CAD build for the part. Positions are in the model's coordinates, mm. A direction names the side the tool comes from. Give positions to 0.01 mm unless a question says otherwise; leave off trailing zeros. Write each loop counter-clockwise with the first axis right and the second up, starting at its lowest first coordinate (ties: lowest second). Pieces come first, ordered by that corner, then holes. Notation, with made-up numbers: (69, 39.25) -> (118, 39.25) arc R21 cw to (118, 46.25) -> close; hole circle Ø11 at (25, 36.5). An arc over 180 degrees is marked (long way). Answer in a Markdown table with one row per item. Add a question column.
```python
from build123d import *

# Parameters (mm, degrees)
BASE_EXTRUDE_DEPTH     = 3.81
SKETCHED_START         = -15.875
SKETCHED_BEND1_DEPTH   = 31.75
SKETCHED_BEND1_2_DEPTH = 31.75


# Read off the part's stored shape, not the designer's step: Sketched Bend1
with BuildPart() as part:
    # Sketch1 → Base-Extrude (new body)
    with BuildSketch(Plane.XY):
        with BuildLine():
            Line((15.875, 68.022105782), (15.875, 254))
            Line((15.875, 254), (-15.875, 254))
            Line((-15.875, 254), (-15.875, 68.022105782))
            ThreePointArc((-15.875, 68.022105782), (0, -69.85), (15.875, 68.022105782))
        make_face()
    extrude(amount=BASE_EXTRUDE_DEPTH)

    # Sketched Bend1 outline → Sketched Bend1 (cut)
    with BuildSketch(Plane.YZ.offset(SKETCHED_START)):
        with BuildLine():
            ThreePointArc((121.7921973, 3.81), (127.40036545, 2.828314461), (132.341609606, 0))
            Line((132.341609606, 0), (254, 0))
            Line((254, 0), (254, 3.81))
            Line((254, 3.81), (121.7921973, 3.81))
        make_face()
    extrude(amount=SKETCHED_BEND1_DEPTH, mode=Mode.SUBTRACT)

    # Sketched Bend1 2 outline → Sketched Bend1 2 (add)
    with BuildSketch(Plane.YZ.offset(SKETCHED_START)):
        with BuildLine():
            Line((123.653365296, -25.262883972), (35.007053077, -38.395670967))
            Line((35.007053077, -38.395670967), (35.565403476, -42.164536159))
            Line((35.565403476, -42.164536159), (124.211715695, -29.031749163))
            ThreePointArc((124.211715695, -29.031749163), (137.690590482, -17.152099982), (132.341609606, 0))
            Line((132.341609606, 0), (121.7921973, 0))
            ThreePointArc((121.7921973, 0), (134.457871906, -11.766894015), (123.653365296, -25.262883972))
        make_face()
    extrude(amount=SKETCHED_BEND1_2_DEPTH)


solid = part.part
```
Item 1: Slice it at C-C, the plane z = -17. List the corners of the cut face in (x, y) (3 decimals), then the cut area to 3 significant figures.
Item 2: Probe L1, parallel to Z at x = 28.5, y = 5.5; L2, parallel to Z at x = -14, y = 50.5; L3, parallel to Z at x = 2.5, y = 73.5. List the from-to ranges inside material, lowest first. Write a range as from..to.
Item 3: Mould opens along Z. For faces 4 (the face through (-0.22, 79.27, -35.69)), 5 (the face through (-0.222, 134.436, -11.502)), 6 (the face through (15.875, 102, -29)) say: released by +Z, released by -Z, zero draft, split by the parting line, or undercut.
Item 4: Slice it at D-D, the plane y = 0. List the corners of the cut face in (x, z).
Item 5: Which spindle directions (+Z, -Z, +X, -X, +Y, -Y) get a long thin tool onto all of the face, cutting with end or side? Do faces 1 (the face through (-15.875, 102, -29)), 2 (the face through (-1, 6, 3.81)), 3 (the face through (-1, 6, 0)). Say none if no direction does.
Item 6: Slice it at A-A, the plane y = 93.5. List the corners of the cut face in (x, z) (3 decimals), then the cut area to 3 significant figures.
Item 7: Slice it at B-B, the plane x = 0. List the corners of the cut face in (y, z), then the cut area to 3 significant figures.
Item 8: Drop flat-ended pins along their axis: pin 1 Ø1.5 at (x, z) = (15.5, -5) entering from -Y; pin 2 Ø3 at (x, y) = (-2.5, 65.5) entering from -Z. Give the stop position or say it passes through.
Answer key:
| question | item | result |
|---|---|---|
| 1 | outline | (-15.875, 133.742) -> (15.875, 133.742) -> (15.875, 137.732) -> (-15.875, 137.732) -> close |
| 1 | area | 127 mm² |
| 2 | L1 | z = 0..3.81 |
| 2 | L2 | z = -39.95..-36.1, 0..3.81 |
| 2 | L3 | z = -36.54..-32.69, 0..3.81 |
| 3 | face 4 | released by -Z |
| 3 | face 5 | undercut |
| 3 | face 6 | zero draft |
| 4 | outline | (-69.85, 0) -> (69.85, 0) -> (69.85, 3.81) -> (-69.85, 3.81) -> close |
| 5 | face 1 | -Z, -X, +Y |
| 5 | face 2 | +Z, +X, -X, +Y, -Y |
| 5 | face 3 | +X, -X, -Y |
| 6 | outline | (-15.875, -33.582) -> (15.875, -33.582) -> (15.875, -29.73) -> (-15.875, -29.73) -> close; (-15.875, 0) -> (15.875, 0) -> (15.875, 3.81) -> (-15.875, 3.81) -> close |
| 6 | area | 243 mm² |
| 7 | outline | (-69.85, 0) -> (121.79, 0) arc R12.7 cw to (123.65, -25.26) -> (35.01, -38.4) -> (35.57, -42.16) -> (124.21, -29.03) arc R16.51 ccw to (121.79, 3.81) -> (-69.85, 3.81) -> close |
| 7 | area | 1,240 mm² |
| 8 | pin 1 | stops at y = 131.27 |
| 8 | pin 2 | stops at z = -37.95 |
